Check sheet for the drawn part. Datum: minimum x, y, z corner. Units: mm. Give positions to 0.01 mm unless a question says otherwise; leave off trailing zeros. Write each loop counter-clockwise with the first axis right and the second up, starting at its lowest first coordinate (ties: lowest second). Pieces come first, ordered by that corner, then holes. Notation, with made-up numbers: (81, -5.75) - (99, -5.75) arc R21 cw to (99, 33.25) - close; hole circle Ø5 at (-24, -39). An arc over 180 degrees is marked (long way). Return JSON: item names as keys, results as strings. Group by question number.
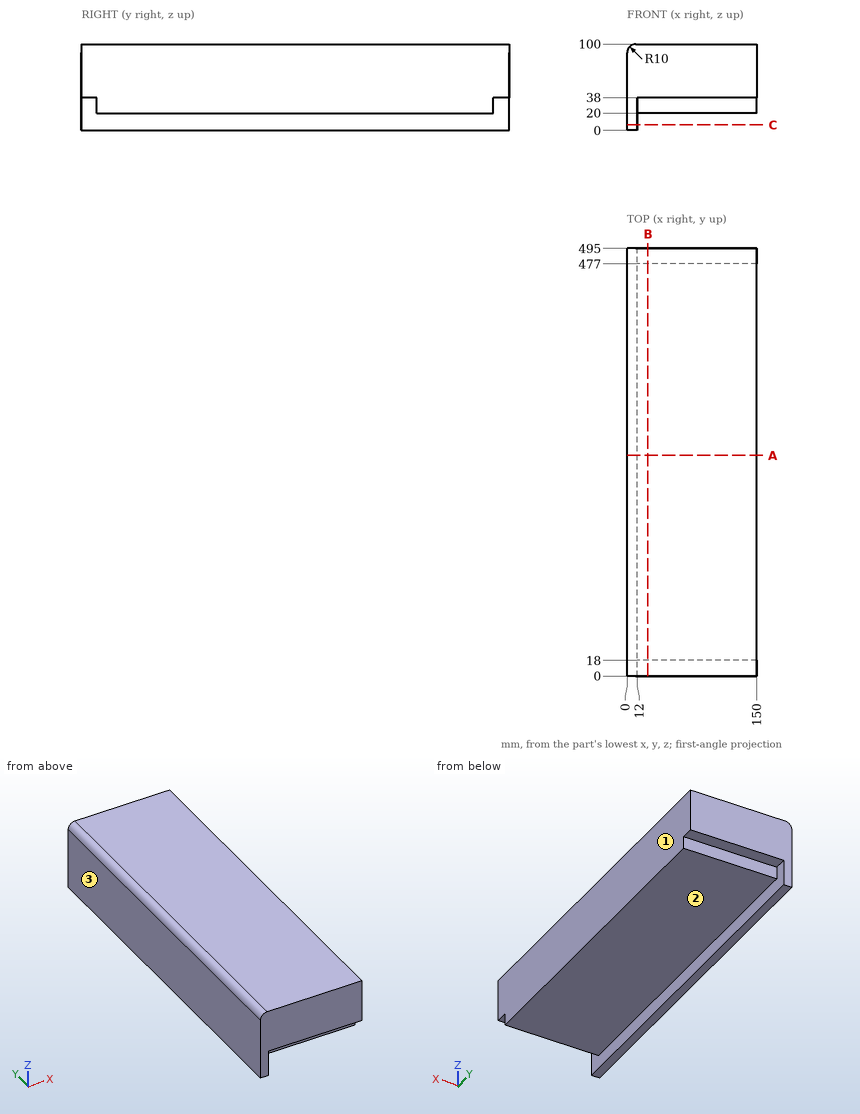
Item 1: Section check A-A on y = 255.5. Record the cut outline in (x, z), plus the area to 3 significant figures.
Item 2: Mould release check, pull along X, two halves, no side actions. Record for the marked faces 1, 2 and 3: +X half, -X half, draft (parallel to the pull), parting line (faces both ways), or undercut.
Item 3: Depth check by flat-ended pin: pin 1 (1 mm diameter, centred on x = 83, y = 310.5, fed in from -Z); pin 2 (3 mm diameter, centred on x = 119, z = 52.5, fed in from -Y); pin 3 (14.5 mm diameter, centred on x = 66.5, z = 30.5, fed in from +Y); pin 4 (14.5 mm diameter, centred on x = 69, z = 28.5, fed in from -Y). Enter the tip coordinate at first touch or a pass-through.
Item 4: Material ranges on line 1 along Z through (x, y) = (50, 292.5); line 2 along Y through (x, z) = (90, 20.5); line 3 along X through (y, z) = (87.5, 14.5), recorded low to high. Write a range as from..to.
Item 5: Section check B-B on x = 24. Record the cut outline in (y, z).
Item 6: Section check C-C on z = 6.5. Record the cut outline in (x, y).
Reply:
{
 "1": {"outline": "(0, 0) - (12, 0) - (12, 20) - (150, 20) - (150, 100) - (10, 100) arc R10 ccw to (0, 90) - close", "area": "12,200 mm²"},
 "2": {"face 1": "+X half", "face 2": "draft", "face 3": "-X half"},
 "3": {"pin 1": "z = 20", "pin 2": "y = 0", "pin 3": "y = 477", "pin 4": "y = 18"},
 "4": {"line 1": "20..100", "line 2": "18..477", "line 3": "0..12"},
 "5": {"outline": "(0, 38) - (18, 38) - (18, 20) - (477, 20) - (477, 38) - (495, 38) - (495, 100) - (0, 100) - close"},
 "6": {"outline": "(0, 0) - (12, 0) - (12, 495) - (0, 495) - close"}
}
